Work out the finished part from the listing and answer in its coordinate system (mm). Coordinates: 2 decimals unless noted, no trailing zeros. Write each loop counter-clockwise with the first axis right and the second up, starting at its lowest first coordinate (ties: lowest second). Pieces come first, ordered by that corner, then holes. Notation, with made-up numbers: (18, -21.5) - (36, -21.5) arc R20 ccw to (36, 11.5) - close; hole circle Ø3 at (62, 23). An arc over 180 degrees is marked (long way). Use a Markdown table: item, result. Add a question column.
(1) The part is cut by section A-A, the plane y = 118.5. Give the vertices of the cut face in (x, z).
(2) The part is cut by section B-B, the plane x = 0. State how many separate pieces and enclosed holes the cut face has, then the cut area to 3 significant figures.
(3) Find the intervals of material crossed by line 1 (X direction, y = 0.5, z = 2.8); line 2 (X direction, y = 19.5, z = 0.5); line 3 (Y direction, x = -7.25, z = 4.05), in increasing order. Write a range as from..to.
(4) Given pin 1 Ø6 at (x, y) = (2, 211) entering from +Z; pin 2 Ø13 at (x, y) = (0, 0) entering from -Z; pin 3 Ø2 at (x, z) = (7, 5.5) entering from -Y; pin 4 Ø3 at (x, z) = (-8, 4) entering from +Y, each flat-ended and moving along its own axis, determine where each tip first touches the part or whether it passes through.
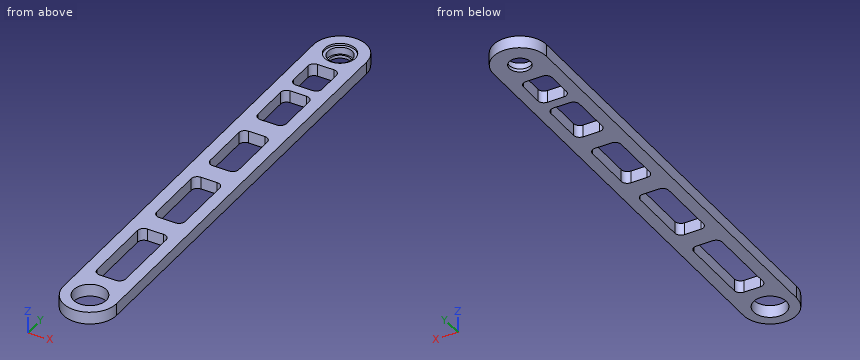
from build123d import *

# Parameters (mm, degrees)
SKETCH_1_R          = 8
EXTRUDE_1_DEPTH     = 6
SKETCH_2_W          = 14
SKETCH_2_H          = 25
SKETCH_2_H_2        = 30
SKETCH_2_H_3        = 35
SKETCH_2_H_4        = 40
SKETCH_2_H_5        = 18
CUT_EXTRUDE_1_DEPTH = 224.45916853
FILLET_1_R          = 3
SKETCH_3_R          = 8
SKETCH_3_R_2        = 5.2
EXTRUDE_2_DEPTH     = 6
SKETCH_4_R          = 6
CUT_EXTRUDE_2_DEPTH = 4.5
SKETCH_5_R          = 7.5
CUT_EXTRUDE_3_DEPTH = 1


with BuildPart() as part:
    # 草图1 → 凸台-拉伸1 (new body)
    with BuildSketch(Plane.XY):
        with BuildLine():
            Line((-13, 0), (-13, 210))
            ThreePointArc((-13, 210), (0, 223), (13, 210))
            Line((13, 210), (13, 0))
            ThreePointArc((13, 0), (0, -13), (-13, 0))
        make_face()
        Circle(SKETCH_1_R, mode=Mode.SUBTRACT)
        with Locations((0, 210)):
            Circle(SKETCH_1_R, mode=Mode.SUBTRACT)
    extrude(amount=EXTRUDE_1_DEPTH)

    # 草图2 → 切除-拉伸1 (cut, through all)
    with BuildSketch(Plane.XY.offset(6)):
        with Locations((0, 162.5)):
            Rectangle(SKETCH_2_W, SKETCH_2_H)
        with Locations((0, 125)):
            Rectangle(SKETCH_2_W, SKETCH_2_H_2)
        with Locations((0, 82.5)):
            Rectangle(SKETCH_2_W, SKETCH_2_H_3)
        with Locations((0, 35)):
            Rectangle(SKETCH_2_W, SKETCH_2_H_4)
        with Locations((0, 189)):
            Rectangle(SKETCH_2_W, SKETCH_2_H_5)
    extrude(amount=-CUT_EXTRUDE_1_DEPTH, mode=Mode.SUBTRACT)

    # 圆角1
    fillet_1_edges = [part.edges().sort_by_distance(p)[0] for p in [
        (7, 140, 3),
        (7, 110, 3),
        (-7, 110, 3),
        (-7, 140, 3),
        (7, 100, 3),
        (7, 65, 3),
        (-7, 65, 3),
        (-7, 100, 3),
        (7, 55, 3),
        (7, 15, 3),
        (-7, 15, 3),
        (-7, 55, 3),
        (7, 198, 3),
        (7, 180, 3),
        (-7, 180, 3),
        (-7, 198, 3),
        (7, 175, 3),
        (7, 150, 3),
        (-7, 150, 3),
        (-7, 175, 3),
    ]]
    fillet(fillet_1_edges, radius=FILLET_1_R)

    # 草图3 → 凸台-拉伸2 (add)
    with BuildSketch(Plane(origin=(0, 0, 0), x_dir=(-1, 0, 0), z_dir=(0, 0, -1))):
        with Locations((0, 210)):
            Circle(SKETCH_3_R)
        with Locations((0, 210)):
            Circle(SKETCH_3_R_2, mode=Mode.SUBTRACT)
    extrude(amount=-EXTRUDE_2_DEPTH)

    # 草图4 → 切除-拉伸2 (cut)
    with BuildSketch(Plane.XY.offset(6)):
        with Locations((0, 210)):
            Circle(SKETCH_4_R)
    extrude(amount=-CUT_EXTRUDE_2_DEPTH, mode=Mode.SUBTRACT)

    # 草图5 → 切除-拉伸3 (cut)
    with BuildSketch(Plane.XY.offset(6)):
        with Locations((0, 210)):
            Circle(SKETCH_5_R)
    extrude(amount=-CUT_EXTRUDE_3_DEPTH, mode=Mode.SUBTRACT)


solid = part.part
Model answer:
| question | item | result |
|---|---|---|
| 1 | outline | (-13, 0) - (-7, 0) - (-7, 6) - (-13, 6) - close; (7, 0) - (13, 0) - (13, 6) - (7, 6) - close |
| 2 | separate pieces | 8 |
| 2 | enclosed holes | 0 |
| 2 | area | 359 mm^2 |
| 3 | line 1 | -13..-7.98, 7.98..13 |
| 3 | line 2 | -13..-7, 7..13 |
| 3 | line 3 | -10.79..-3.38, 3.38..220.79 |
| 4 | pin 1 | z = 1.5 |
| 4 | pin 2 | through |
| 4 | pin 3 | y = -11.53 |
| 4 | pin 4 | y = 221.26 |
